Build history of the part. All positions in model axes, mm. Give positions to 0.01 mm unless a question says otherwise; leave off trailing zeros. Write each loop counter-clockwise with the first axis right and the second up, starting at its lowest first coordinate (ties: lowest second). Pieces come first, ordered by that corner, then holes. Notation, with made-up numbers: M 5.5,55 L 16.5,55 A17 cw 16.5,65 Z; hole C 1.25,82.25 d9. An arc over 180 degrees is marked long. Return JSON: item names as keys, results as strings. Group by question number.
Q1. Band-saw the part on C-C, the plane z = 17.5. Give the cut face in (x, y) (3 decimals).
Q2. Flat gauge pins, fed straight in: pin 1 Ø5 at (y, z) = (-12, 21) entering from +X; pin 2 Ø6 at (y, z) = (-11, 24) entering from +X. Where does each tip first touch, or does it go through?
Q3. Band-saw the part on A-A, the plane x = 556.5. Give the cut face in (y, z) (3 decimals).
Q4. Band-saw the part on B-B, the plane y = -2.5. Give the cut face in (x, z), then the cut area to 3 significant figures.
Q5. Wall check: probe 1 along Y at (x, z) = (1250, 16) (3 decimals); probe 2 along Z at (x, y) = (1231, -6.5); probe 3 along X at (y, z) = (-10, 29.5). Give the ranges that are in metal, low to high.
from build123d import *

# Parameters (mm, degrees)
SKETCH_W        = 31.75
SKETCH_H        = 31.75
SKETCH_W_2      = 26.2128
SKETCH_H_2      = 26.2128
PAD_DEPTH       = 1452.84
POCKET_DEPTH    = 31.75
POCKET001_DEPTH = 31.75


with BuildPart() as part:
    # Sketch → Pad (new body)
    with BuildSketch(Plane.YZ):
        with Locations((0, 15.875)):
            Rectangle(SKETCH_W, SKETCH_H)
        with Locations((0, 15.875)):
            Rectangle(SKETCH_W_2, SKETCH_H_2, mode=Mode.SUBTRACT)
    extrude(amount=PAD_DEPTH)

    # Sketch001 → Pocket (cut)
    with BuildSketch(Plane(origin=(0, -15.875, 0), x_dir=(0, 0, -1), z_dir=(0, -1, 0))):
        Polygon((0, 0), (-31.75, 0), (-31.75, 3.356827), align=None)
    extrude(amount=-POCKET_DEPTH, mode=Mode.SUBTRACT)

    # Sketch002 → Pocket001 (cut)
    with BuildSketch(Plane(origin=(0, -15.875, 0), x_dir=(0, 0, -1), z_dir=(0, -1, 0))):
        Polygon((-31.75, 1452.84), (0, 1452.84), (0, 1449.483173), align=None)
    extrude(amount=-POCKET001_DEPTH, mode=Mode.SUBTRACT)


solid = part.part
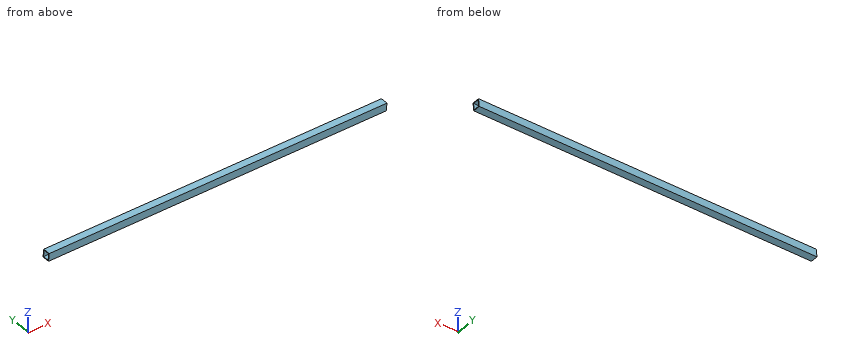
From the geometry:
{
 "1": {"outline": "M 1.85,-15.875 L 1451.333,-15.875 L 1451.333,-13.106 L 1.85,-13.106 Z; M 1.85,13.106 L 1451.333,13.106 L 1451.333,15.875 L 1.85,15.875 Z"},
 "2": {"pin 1": "stops at x = 1451.94", "pin 2": "stops at x = 1452.25"},
 "3": {"outline": "M -15.875,0 L 15.875,0 L 15.875,31.75 L -15.875,31.75 Z; hole M -13.106,2.769 L 13.106,2.769 L 13.106,28.981 L -13.106,28.981 Z"},
 "4": {"outline": "M 0,0 L 1449.48,0 L 1449.78,2.77 L 0.29,2.77 Z; M 3.06,28.98 L 1452.55,28.98 L 1452.84,31.75 L 3.36,31.75 Z", "area": "8,030 mm^2"},
 "5": {"probe 1": "y = -15.875 to -13.106, 13.106 to 15.875", "probe 2": "z = 0 to 2.77, 28.98 to 31.75", "probe 3": "x = 3.12 to 1452.6"}
}
